Can you work these out from the model? Positions are in its coordinate system, mm. A direction names the side the tool comes from. Give positions to 0.01 mm unless a question says otherwise; leave off trailing zeros. Order: outer loops, then holes, each group sorted by start corner. A loop starts at its lowest first (then second) coordinate and runs counter-clockwise, first axis right, second up. Notation, with made-up numbers: M 10.5,-1.5 L 41.5,-1.5 A17 ccw 41.5,6.5 Z; hole C 89,-27 d4. An arc over 180 degrees is marked long. One line per question, with ' | ' between items. Start each with the question number.
1) If we section it at A-A, the plane x = 0: Please give me the cut outline in (y, z).
2) Please list where these lines run through material, in increasing order: line 1 along Z through (x, y) = (0.25, -3.5); line 2 along Z through (x, y) = (0.75, -0.25); line 3 along X through (y, z) = (0, -14.75). Write a range as [from, to].
3) If we section it at B-B, the plane z = -12: Please give me the cut outline in (x, y).
4) I'm going to push flat-ended pins straight in: pin 1 Ø1.5 at (x, z) = (-2, -11) entering from +Y; pin 2 Ø5 at (y, z) = (-2.5, -6.5) entering from -X. Where does each tip first touch, or does it pass through?
5) Thinking about a two-plate mould opening in Y: for faces 4 (the cylindrical face through (2.285, -3.584, -2.468)), 5 (the flat face through (0, 0, -30)), 6 (the flat face through (0, 2, -1)), 7 (the flat face through (-1.724, 1.014, -1.232)), which applies, +Y half, -Y half, draft (parallel to the pull), parting line (faces both ways), or undercut?
6) For faces 1 (the flat face through (-2, 1, 0)), 2 (the flat face through (-2, -2, -5)), 3 (the flat face through (-1.74, -0.99, -1.23)), which set-ups out of +Z, -Z, +X, -X, +Y, -Y let a thin tool reach every point of the face, with its end or its side?
```python
from build123d import *

# Parameters (mm, degrees)
F3_DEPTH = 2.5
F4_SIZE  = 0.5
F5_SIZE  = 0.25


with BuildPart() as f1:
    # F0 (on Front) → F1 (revolve)
    with BuildSketch(Plane.XZ):
        Polygon((4.25, 0), (0, 0), (0, -30), (2.5, -30), (2.5, -5), (4.25, -5), align=None)
    revolve(axis=Axis((0, 0, -15), (0, 0, -1)))

    # F2 (on face) → F3 (cut)
    with BuildSketch(Plane.XY):
        Polygon((1.154701, 2), (-1.154701, 2), (-2.309401, 0), (-1.154701, -2), (1.154701, -2), (2.309401, 0), align=None)
    extrude(amount=-F3_DEPTH, mode=Mode.SUBTRACT)

    # F4
    f4_edges = [f1.edges().sort_by_distance(p)[0] for p in [
        (-2.5, 0, -30),
    ]]
    chamfer(f4_edges, length=F4_SIZE)

    # F5
    f5_edges = [f1.edges().sort_by_distance(p)[0] for p in [
        (-4.25, 0, 0),
        (-4.25, 0, -5),
    ]]
    chamfer(f5_edges, length=F5_SIZE)


solid = f1.part
```
Results found:
1) outline: M -4.25,-4.75 L -4,-5 L -2.5,-5 L -2.5,-29.5 L -2,-30 L 2,-30 L 2.5,-29.5 L 2.5,-5 L 4,-5 L 4.25,-4.75 L 4.25,-0.25 L 4,0 L 2,0 L 2,-2.5 L -2,-2.5 L -2,0 L -4,0 L -4.25,-0.25 Z
2) line 1: z = [-5, 0] | line 2: z = [-30, -2.5] | line 3: x = [-2.5, 2.5]
3) outline: C 0,0 d5
4) pin 1: stops at y = 2.17 | pin 2: stops at x = -4.19
5) face 4: parting line | face 5: draft | face 6: undercut | face 7: undercut
6) face 1: +Z, +X, -X, +Y, -Y | face 2: -Z | face 3: +Z
